```python
from build123d import *

# Parameters (mm, degrees)
BOSS_EXTRUDE1_DEPTH     = 6
SKETCH2_R               = 7.5
BOSS_EXTRUDE2_DEPTH     = 28
BOSS_EXTRUDE3_DEPTH     = 6
SKETCH4_R               = 6.75
CUT_EXTRUDE1_DEPTH      = 49.590122453
CUT_EXTRUDE2_DEPTH      = 49.590122453
CUT_EXTRUDE2_DEPTH_BACK = 49.590122453
SKETCH5_W               = 23
SKETCH5_H               = 3
SKETCH6_R               = 1.75
CUT_EXTRUDE3_DEPTH      = 50.899899799
CHAMFER1_SIZE           = 3


with BuildPart() as part:
    # Sketch1 → Boss-Extrude1 (new body)
    with BuildSketch(Plane.XY):
        with BuildLine():
            Line((-11, 0), (-11, -12))
            Line((-11, -12), (-19, -12))
            Line((-19, -12), (-19, -20))
            Line((-19, -20), (-11, -20))
            Line((-11, -20), (11, -20))
            Line((11, -20), (19, -20))
            Line((19, -20), (19, -12))
            Line((19, -12), (11, -12))
            Line((11, -12), (11, 0))
            ThreePointArc((11, 0), (0, 11), (-11, 0))
        make_face()
    extrude(amount=BOSS_EXTRUDE1_DEPTH)

    # Sketch2 → Boss-Extrude2 (add)
    with BuildSketch(Plane.XY.offset(6)):
        Circle(SKETCH2_R)
    extrude(amount=BOSS_EXTRUDE2_DEPTH)

    # Sketch3 → Boss-Extrude3 (add)
    with BuildSketch(Plane.XY.offset(34)):
        with BuildLine():
            Line((-11, 0), (-11, -12))
            Line((-11, -12), (-19, -12))
            Line((-19, -12), (-19, -20))
            Line((-19, -20), (19, -20))
            Line((19, -20), (19, -12))
            Line((19, -12), (11, -12))
            Line((11, -12), (11, 0))
            ThreePointArc((11, 0), (0, 11), (-11, 0))
        make_face()
    extrude(amount=BOSS_EXTRUDE3_DEPTH)

    # Sketch4 → Cut-Extrude1 (cut, through all)
    with BuildSketch(Plane.XY.offset(40)):
        Circle(SKETCH4_R)
    extrude(amount=-CUT_EXTRUDE1_DEPTH, mode=Mode.SUBTRACT)

    # Sketch5 → Cut-Extrude2 (cut, two sides: drawn at the far end of the back side and taken through both)
    with BuildSketch(Plane(origin=(0, 0, 0), x_dir=(-1, 0, 0), z_dir=(0, 0, -1)).offset(-CUT_EXTRUDE2_DEPTH_BACK)):
        with Locations((0, -18.5)):
            Rectangle(SKETCH5_W, SKETCH5_H)
    extrude(amount=CUT_EXTRUDE2_DEPTH + CUT_EXTRUDE2_DEPTH_BACK, mode=Mode.SUBTRACT)

    # Sketch6 → Cut-Extrude3 (cut, through all)
    with BuildSketch(Plane(origin=(0, -12, 0), x_dir=(1, 0, 0), z_dir=(0, 1, 0))):
        with Locations(Location((-15, -3, 0), (0, 0, 270))):
            Circle(SKETCH6_R)
        with Locations(Location((15, -3, 0), (0, 0, 270))):
            Circle(SKETCH6_R)
        with Locations(Location((15, -37, 0), (0, 0, 270))):
            Circle(SKETCH6_R)
        with Locations(Location((-15, -37, 0), (0, 0, 270))):
            Circle(SKETCH6_R)
    extrude(amount=-CUT_EXTRUDE3_DEPTH, mode=Mode.SUBTRACT)

    # Chamfer1
    chamfer1_edges = [part.edges().sort_by_distance(p)[0] for p in [
        (-11, -6, 0),
        (0, 11, 0),
        (11, -6, 0),
        (11, -6, 40),
        (0, 11, 40),
        (-11, -6, 40),
    ]]
    chamfer(chamfer1_edges, length=CHAMFER1_SIZE)


solid = part.part
```
Model file for the job. Use its own axes, mm. A direction names the side the tool comes from. Coordinates: 2 decimals unless noted, no trailing zeros. Loops run counter-clockwise (first coordinate to the right, second up) from the corner with the lowest first, then second, coordinate; pieces in that order, holes last. Notation, with made-up numbers: M 38.5,78.25 L 96.5,78.25 A21 cw 96.5,107.25 Z; hole C 6.25,-8.75 d7. An arc over 180 degrees is marked long. Use CSV: the item, a comma, the result in double quotes. Start each with the question number.
1. Probe probe 1 along X at (y, z) = (-16.25, 37); probe 2 along X at (y, z) = (-17.25, 37); probe 3 along Z at (x, y) = (-16, -12.5). List the from-to ranges inside material, lowest first. Write a range as [from, to].
2. Flat gauge pins, fed straight in: pin 1 (1.8 mm diameter, centred on x = -4.5, z = 36, fed in from -Y); pin 2 (17.5 mm diameter, centred on x = 0, y = 0, fed in from +Z); pin 3 (2.5 mm diameter, centred on y = -8.5, z = 35.5, fed in from -X); pin 4 (12 mm diameter, centred on y = 1.5, z = 29.5, fed in from +X). Where does each tip first touch, or does it go through?
3. Band-saw the part on A-A, the plane x = 15. List the corners of the cut face in (y, z), then the cut area to 3 significant figures.
4. Band-saw the part on B-B, the plane y = -16. List the corners of the cut face in (x, z).
5. Band-saw the part on D-D, the plane y = -9. List the corners of the cut face in (x, z), then the cut area to 3 significant figures.
6. Band-saw the part on C-C, the plane x = 0. List the corners of the cut face in (y, z).
7. Two-plate mould, pull along X, no slides. Class faces 1 (the flat face through (11.5, -19, 37)), 2 (the flat face through (-10, -6, 38)), 3 (the flat face through (13.6, -12, 1.6)): pulls with the +X half, pulls with the -X half, needs draft (parallel to the pull), parting line crosses it, or undercut.
8. Tool access for faces 4 (the cylindrical face through (-7.493, 0.33, 19.804)), 5 (the flat face through (11, -6, 35)), 6 (the flat face through (-13, -12, 2)): list every direction of +Z, -Z, +X, -X, +Y, -Y with a clear straight run to the whole face (end or side of a thin tool).
Entries:
1,probe 1,"x = [-19, -16.75], [-13.25, 13.25], [16.75, 19]"
1,probe 2,"x = [-19, -16.75], [-13.25, -11.5], [11.5, 13.25], [16.75, 19]"
1,probe 3,"z = [0, 1.56], [4.44, 6], [34, 35.56], [38.44, 40]"
2,pin 1,"stops at y = -17"
2,pin 2,"stops at z = 40"
2,pin 3,"stops at x = -11"
2,pin 4,"stops at x = 11"
3,outline,"M -20,0 L -12,0 L -12,1.25 L -20,1.25 Z; M -20,4.75 L -12,4.75 L -12,6 L -20,6 Z; M -20,34 L -12,34 L -12,35.25 L -20,35.25 Z; M -20,38.75 L -12,38.75 L -12,40 L -20,40 Z"
3,area,"40.0 mm2"
4,outline,"M -19,0 L 19,0 L 19,6 L -19,6 Z; M -19,34 L 19,34 L 19,40 L -19,40 Z; hole C -15,3 d3.5; hole C -15,37 d3.5; hole C 15,3 d3.5; hole C 15,37 d3.5"
5,outline,"M -11,3 L -8,0 L 8,0 L 11,3 L 11,6 L -11,6 Z; M -11,34 L 11,34 L 11,37 L 8,40 L -8,40 L -11,37 Z"
5,area,"246 mm2"
6,outline,"M -17,0 L -6.75,0 L -6.75,40 L -17,40 L -17,34 L -7.5,34 L -7.5,6 L -17,6 Z; M 6.75,0 L 8,0 L 11,3 L 11,6 L 7.5,6 L 7.5,34 L 11,34 L 11,37 L 8,40 L 6.75,40 Z"
7,face 1,"undercut"
7,face 2,"pulls with the -X half"
7,face 3,"needs draft"
8,face 4,"none"
8,face 5,"+Z, -Z, +X, +Y"
8,face 6,"-Z, -X, +Y"
